from build123d import *

# Parameters (mm, degrees)
SKETCH1_W           = 40
SKETCH1_H           = 38
BOSS_EXTRUDE2_DEPTH = 30
SKETCH3_W           = 35
SKETCH3_H           = 33
CUT_EXTRUDE1_DEPTH  = 25
SKETCH4_W           = 35
SKETCH4_H           = 19
CUT_EXTRUDE3_DEPTH  = 30
CUT_EXTRUDE4_START  = -79.225806
SKETCH5_W           = 33.033354951
SKETCH5_H           = 1.733302189
CUT_EXTRUDE4_DEPTH  = 100


with BuildPart() as part:
    # Sketch1 → Boss-Extrude2 (new body)
    with BuildSketch(Plane(origin=(0, 0, 0), x_dir=(1, 0, 0), z_dir=(0, 1, 0))):
        with Locations((0.774193548, -6.419354839)):
            Rectangle(SKETCH1_W, SKETCH1_H)
    extrude(amount=BOSS_EXTRUDE2_DEPTH)

    # Sketch3 → Cut-Extrude1 (cut)
    with BuildSketch(Plane(origin=(0, 0, 0), x_dir=(1, 0, 0), z_dir=(0, 1, 0))):
        with Locations((0.774193548, -6.419354839)):
            Rectangle(SKETCH3_W, SKETCH3_H)
    extrude(amount=CUT_EXTRUDE1_DEPTH, mode=Mode.SUBTRACT)

    # Sketch4 → Cut-Extrude3 (cut)
    with BuildSketch(Plane(origin=(0, 0, 0), x_dir=(1, 0, 0), z_dir=(0, 1, 0))):
        with Locations((0.826342552, -2.919354839)):
            Rectangle(SKETCH4_W, SKETCH4_H)
    extrude(amount=CUT_EXTRUDE3_DEPTH, mode=Mode.SUBTRACT)

    # Sketch5 → Cut-Extrude4 (cut)
    with BuildSketch(Plane(origin=(0, 0, 0), x_dir=(0, 0, -1), z_dir=(1, 0, 0)).offset(CUT_EXTRUDE4_START)):
        with Locations((-6.580047935, 5.546955331)):
            Rectangle(SKETCH5_W, SKETCH5_H)
    extrude(amount=CUT_EXTRUDE4_DEPTH, mode=Mode.SUBTRACT)


solid = part.part
Design review of the part built by this model. Coordinates are the model's own, in mm. A direction names the side the tool comes from. Give positions to 0.01 mm unless a question says otherwise; leave off trailing zeros. Order: outer loops, then holes, each group sorted by start corner. A loop starts at its lowest first (then second) coordinate and runs counter-clockwise, first axis right, second up.
1. Tool access review of faces 1 (the flat face through (0, 15, -12.581)), 2 (the flat face through (-18, 6, -9.937)), 3 (the flat face through (18.274, 16, 18)), 4 (the flat face through (1, 27, -6.581)): name each direction out of +Z, -Z, +X, -X, +Y, -Y from which nothing blocks a thin tool from reaching the whole face with its end or side.
Solution:
face 1: -Z, +X, -X, +Y, -Y
face 2: +X, -X
face 3: -Y
face 4: +Y, -Y
2. For pin 1 Ø6 at (x, z) = (-4, 7) entering from -Y; pin 2 Ø3 at (x, z) = (-7.5, 13) entering from -Y, all flat-tipped, find the tip position at first contact; note any pin that passes through.
Solution:
pin 1: passes through
pin 2: stops at y = 25
3. To check wall thickness, follow L1, parallel to Z at x = 10.5, y = 18.5; L2, parallel to X at y = 14.5, z = 20; L3, parallel to Z at x = 6.5, y = 26. State the ranges of each line that lie inside material, in increasing order.
Solution:
L1: z = -12.58 to -10.08, 22.92 to 25.42
L2: x = -19.23 to -16.73, 18.27 to 20.77
L3: z = -12.58 to -6.58, 12.42 to 25.42
4. Add section C-C, the plane y = 17. State the section outline as (x, z) points, then the cut area to 3 significant figures.
Solution:
outline: (-19.23, -12.58) - (20.77, -12.58) - (20.77, 25.42) - (-19.23, 25.42) - close; hole (-16.73, -10.08) - (18.27, -10.08) - (18.27, -6.58) - (18.33, -6.58) - (18.33, 12.42) - (18.27, 12.42) - (18.27, 22.92) - (-16.73, 22.92) - close
area: 364 mm2
5. Add section B-B, the plane z = 15. State the section outline as (x, y) points.
Solution:
outline: (-19.23, 0) - (-16.73, 0) - (-16.73, 4.68) - (-19.23, 4.68) - close; (-19.23, 6.41) - (-16.73, 6.41) - (-16.73, 25) - (18.27, 25) - (18.27, 6.41) - (20.77, 6.41) - (20.77, 30) - (-19.23, 30) - close; (18.27, 0) - (20.77, 0) - (20.77, 4.68) - (18.27, 4.68) - close
6. Add section A-A, the plane z = -4. State the section outline as (x, y) points, then the cut area to 3 significant figures.
Solution:
outline: (-19.23, 0) - (-16.73, 0) - (-16.73, 4.68) - (-19.23, 4.68) - close; (-19.23, 6.41) - (-16.73, 6.41) - (-16.73, 25) - (-16.67, 25) - (-16.67, 30) - (-19.23, 30) - close; (18.33, 0) - (20.77, 0) - (20.77, 4.68) - (18.33, 4.68) - close; (18.33, 6.41) - (20.77, 6.41) - (20.77, 30) - (18.33, 30) - close
area: 140 mm2
7. Add section D-D, the plane x = -6. State the section outline as (y, z) points.
Solution:
outline: (0, -12.58) - (30, -12.58) - (30, -6.58) - (25, -6.58) - (25, -10.08) - (0, -10.08) - close; (0, 22.92) - (4.68, 22.92) - (4.68, 23.1) - (6.41, 23.1) - (6.41, 22.92) - (25, 22.92) - (25, 12.42) - (30, 12.42) - (30, 25.42) - (0, 25.42) - close
8. Mouldability with a two-part tool opening along X and no side actions: class faces 5 (the flat face through (-19.226, 15, 7)), 6 (the flat face through (1, 25, 14)), 7 (the flat face through (1, 0, -11)) as +X half, -X half, draft (parallel to the pull), parting line (faces both ways), or undercut.
Solution:
face 5: -X half
face 6: undercut
face 7: draft
